from build123d import *

# Parameters (mm, degrees)
BLADE_EXTRUDE_DEPTH        = 10
BLADE_CUT_SIZE             = 1
EDGE_ROUNDING_R            = 1
SKETCH2_R                  = 1
HOLE_FOR_SCREW_BLADE_DEPTH = 10


with BuildPart() as part:
    # Sketch1 → Blade Extrude (new body)
    with BuildSketch(Plane.XY):
        Polygon((20, 0), (-20, 0), (-42.627416998, 22.627416998), (-41.920310217, 23.334523779), (-19.585786438, 1), (19.585786438, 1), (41.920310217, 23.334523779), (42.627416998, 22.627416998), align=None)
    extrude(amount=BLADE_EXTRUDE_DEPTH)

    # Blade Cut
    blade_cut_edges = [part.edges().sort_by_distance(p)[0] for p in [
        (30.753048327, 12.16726189, 0),
        (-30.753048327, 12.16726189, 10),
    ]]
    chamfer(blade_cut_edges, length=BLADE_CUT_SIZE - 0.0001)  # a hair under: the kernel refuses the full size

    # Edge Rounding
    edge_rounding_edges = [part.edges().sort_by_distance(p)[0] for p in [
        (20.292822508, 1, 0.49995),
        (-20.292822508, 1, 9.50005),
    ]]
    fillet(edge_rounding_edges, radius=EDGE_ROUNDING_R)

    # Sketch2 → Hole for Screw (Blade) (cut)
    with BuildSketch(Plane(origin=(0, 1, 0), x_dir=(1, 0, 0), z_dir=(0, 1, 0))):
        with Locations(Location((0, -5, 0), (0, 0, 180))):
            Circle(SKETCH2_R)
    extrude(amount=-HOLE_FOR_SCREW_BLADE_DEPTH, mode=Mode.SUBTRACT)


solid = part.part
Geometry: final body of the model. Coordinates: model frame, mm. A direction names the side the tool comes from. Give positions to 0.01 mm unless a question says otherwise; leave off trailing zeros. Order: outer loops, then holes, each group sorted by start corner. A loop starts at its lowest first (then second) coordinate and runs counter-clockwise, first axis right, second up. Notation, with made-up numbers: (-1.5, 60) -> (19.5, 60) arc R18 ccw to (19.5, 89) -> close; hole circle Ø1 at (-38.75, 83.5). An arc over 180 degrees is marked (long way). Put each result on its own line as item: value.
Q1. Draft query along X for faces 4 (the face through (-30.909, 12.324, 3.707)), 5 (the face through (31, 11, 5)), 6 (the face through (0.3, 0, 3.8)). Return one class per face: released by +X, released by -X, zero draft, split by the parting line, or undercut.
Here are the results:
face 4: undercut
face 5: released by +X
face 6: zero draft
Q2. Section D-D, the plane x = 9. Return loops of the section in (y, z).
Here are the results:
outline: (0, 0) -> (1, 0) -> (1, 10) -> (0, 10) -> close
Q3. Section A-A, the plane z = 5. Return loops of the section in (x, y), then the cut area to 3 significant figures.
Here are the results:
outline: (-42.63, 22.63) -> (-20, 0) -> (-1, 0) -> (-1, 1) -> (-19.59, 1) -> (-41.92, 23.33) -> close; (1, 0) -> (20, 0) -> (42.63, 22.63) -> (41.92, 23.33) -> (19.59, 1) -> (1, 1) -> close
area: 101 mm^2
Q4. Reachability of faces 1 (the face through (31.209, 11.906, 0.493)), 2 (the face through (30.597, 12.011, 5.078)), 3 (the face through (-31.514, 12.212, 9.507)) from +Z, -Z, +X, -X, +Y, -Y: full face, straight path, thin tool, end or side. Return the list, or none.
Here are the results:
face 1: -Z, +Y
face 2: +Z, -Z, +Y
face 3: +Z, +Y
Q5. Pin query (flat end, axial travel): pin 1 (4 mm diameter, centred on x = -16.5, z = 7.5, fed in from +Y); pin 2 (5 mm diameter, centred on y = 19, z = 4.5, fed in from -X). Return the tip coordinate at first contact, or that it passes through.
Here are the results:
pin 1: stops at y = 1
pin 2: stops at x = -41.5
Q6. Section B-B, the plane x = 0. Return loops of the section in (y, z), then the cut area to 3 significant figures.
Here are the results:
outline: (0, 0) -> (1, 0) -> (1, 4) -> (0, 4) -> close; (0, 6) -> (1, 6) -> (1, 10) -> (0, 10) -> close
area: 8.00 mm^2
Q7. Material intervals for L1, parallel to Z at x = 0, y = 0.3; L2, parallel to Y at x = 17, z = 3.75; L3, parallel to X at y = 14.25, z = 3, sorted ascending.
Here are the results:
L1: z = 0 to 4, 6 to 10
L2: y = 0 to 1
L3: x = -34.25 to -32.84, 32.84 to 34.25
